CAD build for the part. Positions are in the model's coordinates, mm. A direction names the side the tool comes from. Round coordinates to 2 decimals unless told otherwise and drop trailing zeros. Loops run counter-clockwise (first coordinate to the right, second up) from the corner with the lowest first, then second, coordinate; pieces in that order, holes last. Notation, with made-up numbers: M 25.25,82 L 64.25,82 A24 cw 64.25,106 Z; hole C 44,25.5 d4. An arc over 180 degrees is marked long. Put each result on its own line as item: value. Start each with the question number.
from build123d import *

# Parameters (mm, degrees)
F1_DEPTH = 30
F2_R     = 17.5
F2_R_2   = 10
F3_DEPTH = 64
F4_DEPTH = 32.001
F5_W     = 35
F5_H     = 20
F6_DEPTH = 93


with BuildPart() as f1:
    # F0 (on Front) → F1 (new body, symmetric)
    with BuildSketch(Plane.XZ):
        Polygon((0, 0.2733823939), (-30, 0.2733823939), (-30, -31.7266176061), (-17.5, -31.7266176061), (-17.5, -11.7266176061), (0, -11.7266176061), (17.5, -11.7266176061), (17.5, -31.7266176061), (30, -31.7266176061), (30, 0.2733823939), align=None)
    extrude(amount=F1_DEPTH, both=True)

    # F2 (on face) → F3 (join)
    with BuildSketch(Plane.XY.offset(0.2733823939)):
        Circle(F2_R)
        Circle(F2_R_2, mode=Mode.SUBTRACT)
    extrude(amount=F3_DEPTH)

    # F4 (cut, through all): a face of the model
    f4_faces = [f1.faces().sort_by_distance(p)[0] for p in [
        (0, 0, 0.2733823939),
    ]]
    extrude(f4_faces, amount=-F4_DEPTH, mode=Mode.SUBTRACT)

    # F5 (on face) → F6 (cut)
    with BuildSketch(Plane(origin=(-30, 0, 0), x_dir=(0, -1, 0), z_dir=(-1, 0, 0))):
        with Locations((0, -21.7266176061)):
            Rectangle(F5_W, F5_H)
    extrude(amount=-F6_DEPTH, mode=Mode.SUBTRACT)


solid = f1.part
(1) Cut at B-B on x = 0. List the corners of the cut face in (y, z), and give its area (3 significant figures).
(2) Tool access for faces 4 (the cylindrical face through (-13.887, -10.648, 31.825)), 5 (the flat face through (0, -30, -8)), 6 (the flat face through (24, -17.5, -22)), 7 (the flat face through (24, 24, -31.727)), 8 (the flat face through (17.5, -24, -22)): list every direction of +Z, -Z, +X, -X, +Y, -Y with a clear straight run to the whole face (end or side of a thin tool).
(3) Cut at D-D on x = 23. List the corners of the cut face in (y, z).
(4) Cut at A-A on z = -21.5. List the corners of the cut face in (x, y), and give its area (3 significant figures).
(5) Drill centre lines: line 1 along Y through (x, z) = (0, 15); line 2 along Z through (x, y) = (22, 19); line 3 along Y through (x, z) = (4, -4). Where is each one in solid material? Low to high.
(6) Flat gauge pins, fed straight in: pin 1 Ø18 at (x, y) = (13, -14.5) entering from +Z; pin 2 Ø4 at (x, y) = (-13, 17) entering from -Z; pin 3 Ø1.5 at (x, z) = (-3, 19) entering from -Y; pin 4 Ø3 at (y, z) = (-16, 7.5) entering from +X. Where does each tip first touch, or does it go through?
(7) Mould opens along X. For faces 1 (the flat face through (-17.5, -24, -22)), 2 (the flat face through (24, 17.5, -22)), 3 (the flat face through (30, 0, -9)) say: +X half, -X half, draft (parallel to the pull), parting line (faces both ways), or undercut.
Taken from the geometry:
1. outline: M -30,-11.73 L -10,-11.73 L -10,64.27 L -17.5,64.27 L -17.5,0.27 L -30,0.27 Z; M 10,-11.73 L 30,-11.73 L 30,0.27 L 17.5,0.27 L 17.5,64.27 L 10,64.27 Z
1. area: 1,440 mm2
2. face 4: +Z
2. face 5: +Z, -Z, +X, -X, -Y
2. face 6: -Z, +X, -X
2. face 7: -Z, +X, -X, +Y, -Y
2. face 8: -Z, +Y, -Y
3. outline: M -30,-31.73 L -17.5,-31.73 L -17.5,-11.73 L 17.5,-11.73 L 17.5,-31.73 L 30,-31.73 L 30,0.27 L -30,0.27 Z
4. outline: M -30,-30 L -17.5,-30 L -17.5,-17.5 L -30,-17.5 Z; M -30,17.5 L -17.5,17.5 L -17.5,30 L -30,30 Z; M 17.5,-30 L 30,-30 L 30,-17.5 L 17.5,-17.5 Z; M 17.5,17.5 L 30,17.5 L 30,30 L 17.5,30 Z
4. area: 625 mm2
5. line 1: -17.5 to -10, 10 to 17.5
5. line 2: -31.73 to 0.27
5. line 3: -30 to -9.17, 9.17 to 30
6. pin 1: z = 64.27
6. pin 2: z = -11.73
6. pin 3: y = -17.35
6. pin 4: x = 9.8
7. face 1: undercut
7. face 2: draft
7. face 3: +X half
